```python
from build123d import *

# Parameters (mm, degrees)
SKETCH1_R           = 25.4
BOSS_EXTRUDE1_DEPTH = 9.525


with BuildPart() as part:
    # Sketch1 → Boss-Extrude1 (new, symmetric)
    with BuildSketch(Plane.XY):
        Circle(SKETCH1_R)
        with BuildLine():
            Line((1.439619435, 0.51806938), (1.161846601, 0.633255459))
            Line((1.161846601, 0.633255459), (-0.372765644, 1.269624265))
            Line((-0.372765644, 1.269624265), (-0.650538478, 1.384810344))
            ThreePointArc((-0.650538478, 1.384810344), (-1.106507953, 1.056664634), (-1.413303873, 0.586064982))
            ThreePointArc((-1.413303873, 0.586064982), (-0.586064982, -1.413303873), (1.413303873, -0.586064982))
            ThreePointArc((1.413303873, -0.586064982), (1.529565632, -0.036455146), (1.439619435, 0.51806938))
        make_face(mode=Mode.SUBTRACT)
    extrude(amount=BOSS_EXTRUDE1_DEPTH, both=True)


solid = part.part
```
The model under review builds one solid part; all positions refer to its coordinate system, in mm. Round coordinates to 2 decimals unless told otherwise and drop trailing zeros. Write each loop counter-clockwise with the first axis right and the second up, starting at its lowest first coordinate (ties: lowest second). Pieces come first, ordered by that corner, then holes. Notation, with made-up numbers: (-13.75, 2) -> (29.25, 2) arc R12 ccw to (29.25, 12) -> close; hole circle Ø2 at (38.25, -13). An arc over 180 degrees is marked (long way). Use CSV: the item, a comma, the result in double quotes.
Q1. Consider section B-B (x = 16). Give the boundary of the cut face in (y, z) (3 decimals), then the cut area to 3 significant figures.
Checks:
outline,"(-19.727, -9.525) -> (19.727, -9.525) -> (19.727, 9.525) -> (-19.727, 9.525) -> close"
area,"752 mm²"
Q2. Mouldability with a two-part tool opening along X and no side actions: class faces 1 (the cylindrical face through (-5.506, -24.796, 0.133)), 2 (the flat face through (5, 0, -9.525)) as released by +X, released by -X, zero draft, split by the parting line, or undercut.
Checks:
face 1,"split by the parting line"
face 2,"zero draft"
Q3. For pin 1 Ø3 at (y, z) = (-8, 4) entering from +X; pin 2 Ø2 at (x, z) = (6.5, 5.5) entering from +Y; pin 3 Ø6 at (x, z) = (18, 7) entering from +Y, all flat-tipped, find the tip position at first contact; note any pin that passes through.
Checks:
pin 1,"x = 24.55"
pin 2,"y = 24.8"
pin 3,"y = 20.5"
Q4. To check wall thickness, follow probe 1 along Y at (x, z) = (0, -3.25); probe 2 along X at (y, z) = (-2.5, 8.75); probe 3 along X at (y, z) = (3, -5.75). State the ranges of each line that lie inside material, in increasing order. Write a range as [from, to].
Checks:
probe 1,"[-25.4, -1.53], [1.12, 25.4]"
probe 2,"[-25.28, 25.28]"
probe 3,"[-25.22, 25.22]"
Q5. Consider section C-C (y = 4.5). Give the boundary of the cut face in (x, z) (3 decimals), then the cut area to 3 significant figures.
Checks:
outline,"(-24.998, -9.525) -> (24.998, -9.525) -> (24.998, 9.525) -> (-24.998, 9.525) -> close"
area,"952 mm²"
Q6. Consider section A-A (z = -7). Give the boundary of the cut face in (x, y), then the cut area to 3 significant figures.
Checks:
outline,"circle Ø50.8 at (0, 0); hole (-0.65, 1.38) arc R1.53 ccw (long way) to (1.44, 0.52) -> close"
area,"2,020 mm²"
